The model under review builds one solid part; all positions refer to its coordinate system, in mm. A direction names the side the tool comes from. Coordinates: 2 decimals unless noted, no trailing zeros. Write each loop counter-clockwise with the first axis right and the second up, starting at its lowest first coordinate (ties: lowest second). Pieces come first, ordered by that corner, then holes. Notation, with made-up numbers: M 8,48 L 27,48 A6 ccw 27,56 Z; hole C -24.75,84.25 d3. An arc over 180 degrees is marked long. Answer as CSV lines item,"result". Start each with the question number.
Autodesk Inventor part; units mm, degrees
ref_plane "YZ Plane" through (0, 0, 0) normal (1, 0, 0) x (0, 1, 0)
ref_plane "XZ Plane" through (0, 0, 0) normal (0, 1, 0) x (-1, 0, 0)
ref_plane "XY Plane" through (0, 0, 0) normal (0, 0, 1) x (1, 0, 0)
sketch "Sketch1" plane through (0, 0, 0) normal (1, 0, 0) x (0, 1, 0)
  line L0 (0, 0) -> (0, 55.5774) construction
  line L1 (18, -2) -> (18, 16)
  line L2 (23.9, 42.5) -> (26.15, 42.5)
  line L3 (26.15, 42.5) -> (26.15, 45)
  line L4 (26.15, 45) -> (37.5, 45)
  line L5 (37.5, 45) -> (37.5, 42.767)
  line L6 (37.5, 42.767) -> (29.6625, 39.9)
  line L7 (27.9, 35.9) -> (22, 16)
  line L8 (22, 4) -> (29.9, 4)
  line L9 (29.9, 4) -> (29.9, 0)
  line L10 (29.9, 0) -> (20, 0)
  line L11 (20, 0) -> (20, -2)
  line L12 (20, -2) -> (18, -2)
  line L13 (22, 4) -> (22, 16)
  line L14 (29.6625, 39.9) -> (27.9, 39.9)
  line L15 (27.9, 39.9) -> (27.9, 35.9)
  line L16 (23.9, 42.5) -> (23.9, 35.9)
  line L17 (18, 16) -> (23.9, 35.9)
  dimension "d0" = 40
  dimension "d1" = 2
  dimension "d2" = 2
  dimension "d4" = 59.8
  dimension "d5" = 4
  dimension "d7" = 12
  dimension "d8" = 4
  dimension "d9" = 75
  dimension "d10" = 2.233
  dimension "d11" = 52.3
  dimension "d12" = 47.8
  dimension "d13" = 59.325
  dimension "d14" = 5.1
  dimension "d15" = 2.5
  dimension "d16" = 4
  dimension "d17" = 45
revolve "Revolution1" add sketch "Sketch1" angle 360 about axis through (0, 0, 0) along (0, 0, 1)
sketch "Sketch2" plane through (0, 0, 4) normal (0, 0, 1) x (1, 0, 0)
  line L0 (-19.0919, 19.0919) -> (19.0919, 19.0919)
  line L1 (19.0919, 19.0919) -> (19.0919, -19.0919)
  line L2 (19.0919, -19.0919) -> (-19.0919, -19.0919)
  line L3 (-19.0919, -19.0919) -> (-19.0919, 19.0919)
  line L4 (-19.0919, 19.0919) -> (19.0919, -19.0919) construction
  line L5 (19.0919, 19.0919) -> (-19.0919, -19.0919) construction
  point P0 (0, 0)
  dimension "d19" = 54
hole "Hole1" at (-19.0919, 19.0919, 4) at (19.0919, 19.0919, 4) at (-19.0919, -19.0919, 4) at (19.0919, -19.0919, 4) direction (0, 0, -1) diameter 3.4 end through all
properties part number "014" material "Aluminum 6061"
1) To check wall thickness, follow line 1 (X direction, y = 0, z = 8); line 2 (Y direction, x = 0, z = 2); line 3 (Z direction, x = -13, y = 26). State the ranges of each line that lie inside material, in increasing order. Write a range as [from, to].
2) Take a section at C-C on z = 29. Give the boundary of the cut face in (x, y), and give its area (3 significant figures).
3) Clearance check with flat-ended pins moving along their axes: pin 1 Ø8 at (x, z) = (-8, 15) entering from -Y; pin 2 Ø10 at (y, z) = (6.5, 12.5) entering from -X; pin 3 Ø6 at (x, z) = (5.5, 26) entering from +Y. State where each tip first meets the part, or that it passes through.
4) Mouldability with a two-part tool opening along Y and no side actions: class faces 1 (the flat face through (-20.4, -0.4, 0)), 2 (the cylindrical face through (37.18, -4.88, 43.87)), 3 (the cylindrical face through (20.6, 18.31, 1.97)), 4 (the cylindrical face through (20.15, 12.85, 39.15)) as +Y half, -Y half, draft (parallel to the pull), parting line (faces both ways), or undercut.
5) Tool access review of faces 5 (the flat face through (8, -26, 45)), 6 (the cylindrical face through (20.75, -18.72, 1.97)), 7 (the cylindrical face through (25.528, -5.669, 43.768)), 8 (the flat face through (-3, -18, -2)), 9 (the flat face through (20, -20, 39.9)): name each direction out of +Z, -Z, +X, -X, +Y, -Y from which nothing blocks a thin tool from reaching the whole face with its end or side.
Results:
1,line 1,"x = [-22, -18], [18, 22]"
1,line 2,"y = [-29.9, -18], [18, 29.9]"
1,line 3,"z = [0, 4], [39.9, 45]"
2,outline,"C 0,0 d51.71; hole C 0,0 d43.71"
2,area,"600 mm²"
3,pin 1,"stops at y = -21.95"
3,pin 2,"stops at x = -21.95"
3,pin 3,"stops at y = 25.42"
4,face 1,"draft"
4,face 2,"parting line"
4,face 3,"undercut"
4,face 4,"undercut"
5,face 5,"+Z, +X, -X, +Y, -Y"
5,face 6,"-Z"
5,face 7,"+Z"
5,face 8,"-Z, +X, -X, +Y, -Y"
5,face 9,"none"
